```python
from build123d import *
from build123d.topology import SkipClean

# Parameters (mm, degrees)
RESSALTO_EXTRUS_O1_DEPTH    = 1.25
ESBO_O2_R                   = 2.75
CORTE_EXTRUS_O1_DEPTH       = 343.874678981
CONVERTER_S_LIDO1_START     = -1.75
CONVERTER_S_LIDO1_OUTLINE_R = 2.75
CONVERTER_S_LIDO1_DEPTH     = 0.5
RESSALTO_EXTRUS_O2_DEPTH    = 24


# Read off the part's stored shape, not the designer's step: Converter-Sólido1
with BuildPart() as part:
    # Esboço1 → Ressalto-extrusão1 (new, symmetric)
    with BuildSketch(Plane.XY):
        with BuildLine():
            Line((9.781555201, 0), (114.888726767, 0))
            ThreePointArc((114.888726767, 0), (122.038034046, -3.008047095), (124.886250727, -10.222518914))
            ThreePointArc((124.886250727, -10.222518914), (91.45004484, -172.337167523), (2.728289048, -312.078318252))
            ThreePointArc((2.728289048, -312.078318252), (-0.303175893, -314.310106116), (-3.944968584, -315.262997906))
            Line((-3.944968584, -315.262997906), (-64.334809895, -319.288987326))
            ThreePointArc((-64.334809895, -319.288987326), (-71.831840855, -316.613597697), (-75, -309.311135748))
            Line((-75, -309.311135748), (-75, -169.484512567))
            ThreePointArc((-75, -169.484512567), (-74.144640734, -165.437841608), (-71.72489083, -162.083442149))
            ThreePointArc((-71.72489083, -162.083442149), (-20.715574655, -92.974656039), (-0.208905725, -9.563318777))
            ThreePointArc((-0.208905725, -9.563318777), (2.866600834, -2.776191717), (9.781555201, 0))
        make_face()
    extrude(amount=RESSALTO_EXTRUS_O1_DEPTH, both=True)

    # Esboço2 → Corte-extrusão1 (cut, through all)
    with BuildSketch(Plane.XY.offset(1.25)):
        with Locations((93.886250727, -16)):
            Circle(ESBO_O2_R)
    extrude(amount=-CORTE_EXTRUS_O1_DEPTH, mode=Mode.SUBTRACT)

    # Converter-Sólido1 outline → Converter-Sólido1 (add)
    with BuildSketch(Plane.XY.offset(CONVERTER_S_LIDO1_START)):
        with BuildLine():
            ThreePointArc((2.728289048, -312.078318252), (91.45004484, -172.337167523), (124.886250727, -10.222518914))
            ThreePointArc((124.886250727, -10.222518914), (122.038034046, -3.008047095), (114.888726767, 0))
            Line((114.888726767, 0), (9.781555201, 0))
            ThreePointArc((9.781555201, 0), (2.866600835, -2.776191716), (-0.208905725, -9.563318777))
            ThreePointArc((-0.208905725, -9.563318777), (-20.715574655, -92.974656038), (-71.72489083, -162.083442149))
            ThreePointArc((-71.72489083, -162.083442149), (-74.144640734, -165.437841608), (-75, -169.484512567))
            Line((-75, -169.484512567), (-75, -309.311135748))
            ThreePointArc((-75, -309.311135748), (-71.831840855, -316.613597697), (-64.334809895, -319.288987326))
            Line((-64.334809895, -319.288987326), (-3.944968584, -315.262997906))
            ThreePointArc((-3.944968584, -315.262997906), (-0.303175894, -314.310106116), (2.728289048, -312.078318252))
        make_face()
        with Locations((93.886250727, -16)):
            Circle(CONVERTER_S_LIDO1_OUTLINE_R, mode=Mode.SUBTRACT)
    extrude(amount=CONVERTER_S_LIDO1_DEPTH)

    # Esboço8 → Ressalto-extrusão2 (add)
    with SkipClean():  # the faces are left unmerged after this step: merging them gives an invalid solid
        with BuildSketch(Plane(origin=(0, 0, -1.75), x_dir=(-1, 0, 0), z_dir=(0, 0, -1))):
            with BuildLine():
                Line((-118.871838966, -32), (-123.884147664, -32))
                ThreePointArc((-123.884147664, -32), (-97.937341323, -155.347298973), (-39.44403165, -267))
                Line((-39.44403165, -267), (-33.282417311, -267))
                ThreePointArc((-33.282417311, -267), (-92.563373986, -155.504460627), (-118.871838966, -32))
            make_face()
        extrude(amount=-RESSALTO_EXTRUS_O2_DEPTH)


solid = part.part
```
Model file for the job. Use its own axes, mm. A direction names the side the tool comes from. Give positions to 0.01 mm unless a question says otherwise; leave off trailing zeros. Write each loop counter-clockwise with the first axis right and the second up, starting at its lowest first coordinate (ties: lowest second). Pieces come first, ordered by that corner, then holes. Notation, with made-up numbers: M 38.5,74 L 68.5,74 A33 cw 68.5,102 Z; hole C 24,-8 d5. An arc over 180 degrees is marked long. Use a Markdown table: item, result.
1) Cut at A-A (y = -46). List the corners of the cut face in (x, z), and give its area (3 significant figures).
Responses:
| item | result |
|---|---|
| outline | M -4.89,-1.75 L 122.69,-1.75 L 122.69,22.25 L 117.67,22.25 L 117.67,1.25 L -4.89,1.25 Z |
| area | 488 mm2 |
2) Pin check, flat tips, straight feed: pin 1 (9 mm diameter, centred on x = 93.89, y = -16, fed in from +Z); pin 2 (5 mm diameter, centred on x = 60.5, z = 10.5, fed in from -Y); pin 3 (10 mm diameter, centred on x = 84, z = 18.5, fed in from -Y). Stop position of each tip, or through.
Responses:
| item | result |
|---|---|
| pin 1 | stops at z = 1.25 |
| pin 2 | stops at y = -238.89 |
| pin 3 | stops at y = -200.37 |
3) Cut at D-D (y = -87). List the corners of the cut face in (x, z).
Responses:
| item | result |
|---|---|
| outline | M -18.02,-1.75 L 116.69,-1.75 L 116.69,22.25 L 111.59,22.25 L 111.59,1.25 L -18.02,1.25 Z |
4) Cut at B-B (z = 18.5). List the corners of the cut face in (x, y).
Responses:
| item | result |
|---|---|
| outline | M 33.28,-267 L 39.44,-267 A459.4 ccw 123.88,-32 L 118.87,-32 A454.4 cw Z |
5) Drill centre lines: line 1 (Z direction, x = 46.5, y = -127.5); line 2 (X direction, y = -52, z = 18.75); line 3 (X direction, y = -176, z = 20). Where is each one in solid material? Low to high. Write a range as from..to.
Responses:
| item | result |
|---|---|
| line 1 | z = -1.75..1.25 |
| line 2 | x = 117.01..122.05 |
| line 3 | x = 84.53..89.95 |
6) Cut at C-C (x = 57.5). List the corners of the cut face in (y, z), and give its area (3 significant figures).
Responses:
| item | result |
|---|---|
| outline | M -239.71,-1.75 L 0,-1.75 L 0,1.25 L -229.99,1.25 L -229.99,22.25 L -239.71,22.25 Z |
| area | 923 mm2 |
7) Tool access for faces 1 (the cylindrical face through (91.953, -157.17, 11.603)), 2 (the flat face through (92, -158, 22.25)), 3 (the flat face through (36, -267, 12)): list every direction of +Z, -Z, +X, -X, +Y, -Y with a clear straight run to the whole face (end or side of a thin tool).
Responses:
| item | result |
|---|---|
| face 1 | +Z, -X, +Y |
| face 2 | +Z, +X, -X, +Y, -Y |
| face 3 | +Z, +X, -X, -Y |
